from build123d import *

# Parameters (mm, degrees)
F1_DEPTH = 5
F2_D     = 4
F3_R     = 4.9999


# Not quite as in the source:
# - a fillet or chamfer is up to 0.001 mm smaller than in the source, because OpenCascade refuses the exact size
# - ends of sketch curves that miss each other by under 0.0002 mm in the source are joined


with BuildPart() as f1:
    # F0 (on Top) → F1 (new body)
    with BuildSketch(Plane.XY):
        with BuildLine():
            Line((-35, 2.1762e-06), (-35, -35))
            Line((-35, -35), (-27, -35))
            Line((-27, -35), (-27, -22.2710574513))
            ThreePointArc((-27, -22.2710574513), (-32.9393385518, -11.8321585422), (-35, 2.1762e-06))
        make_face()
        with BuildLine():
            Line((-27, -22.2710574513), (-27, -35))
            Line((-27, -35), (0, -35))
            ThreePointArc((0, -35), (-14.9250291324, -31.658229663), (-27, -22.2710574513))
        make_face()
        with BuildLine():
            add(Edge.make_bspline(
                [(0, 45), (-20.1986748725, 45), (-35, 20.0504870868), (-35, 2.1762e-06)],
                knots=[0, 0, 0, 0, 57.0087695372, 57.0087695372, 57.0087695372, 57.0087695372], degree=3))
            ThreePointArc((-35, 2.1762e-06), (-28.4666369261, 20.3629708568), (-11.3056830814, 33.1237306181))
            add(Edge.make_bspline(
                [(0, 37), (-0.2833414452, 37.0069688983), (-1.1232932293, 37.0068386903), (-2.7957299856, 36.8864035146), (-4.9942322029, 36.3521195303), (-7.6997383876, 35.2871018647), (-9.7958540485, 34.148638444), (-11.0540635502, 33.3003360386), (-11.3056830814, 33.1237306181)],
                knots=[0, 0, 0, 0, 0.8506820357, 2.5185967411, 5.0181648841, 7.6012051941, 11.2266191262, 12.1476935207, 12.1476935207, 12.1476935207, 12.1476935207], degree=3))
            add(Edge.make_bspline(
                [(0, 37), (0.2833414452, 37.0069688983), (1.1232932293, 37.0068386903), (2.7957299856, 36.8864035146), (4.9942322029, 36.3521195303), (7.6997383876, 35.2871018647), (9.7958540485, 34.148638444), (11.0540635502, 33.3003360386), (11.3056830814, 33.1237306181)],
                knots=[0, 0, 0, 0, 0.8506820357, 2.5185967411, 5.0181648841, 7.6012051941, 11.2266191262, 12.1476935207, 12.1476935207, 12.1476935207, 12.1476935207], degree=3))
            ThreePointArc((11.3056830814, 33.1237306181), (28.4666375592, 20.3629699719), (35, 0))
            add(Edge.make_bspline(
                [(0, 45), (20.1986748725, 45), (35, 20.0504870868), (35, 0)],
                knots=[0, 0, 0, 0, 57.0087695372, 57.0087695372, 57.0087695372, 57.0087695372], degree=3))
        make_face()
        with BuildLine():
            ThreePointArc((-11.3056830814, 33.1237306181), (-28.4666369261, 20.3629708568), (-35, 2.1762e-06))
            ThreePointArc((-35, 2.1762e-06), (-32.9393385518, -11.8321585422), (-27, -22.2710574513))
            Line((-27, -22.2710574513), (-27, 2.1762e-06))
            add(Edge.make_bspline(
                [(-11.3056830814, 33.1237306181), (-12.4097508436, 32.3488132243), (-15.1414824386, 30.0752135158), (-18.8876274503, 25.5283101279), (-22.422035633, 19.604279738), (-25.0662594291, 13.1120426553), (-26.6478130576, 7.1844788974), (-27.0173066601, 2.7756083867), (-27.018694794, 0.6711028041), (-27, 2.1762e-06)],
                knots=[12.1476935207, 12.1476935207, 12.1476935207, 12.1476935207, 16.189226149, 22.7543847852, 29.7183326598, 36.8091409701, 43.7289829573, 48.0262708445, 50.0404462243, 50.0404462243, 50.0404462243, 50.0404462243], degree=3))
        make_face()
        with BuildLine():
            ThreePointArc((27, -22.2710574513), (14.9250291324, -31.658229663), (0, -35))
            Line((0, -35), (27, -35))
            Line((27, -35), (27, -22.2710574513))
        make_face()
        with BuildLine():
            ThreePointArc((-27, -22.2710574513), (-14.9250291324, -31.658229663), (0, -35))
            ThreePointArc((0, -35), (14.9250291324, -31.658229663), (27, -22.2710574513))
            Line((27, -22.2710574513), (27, 2.1762e-06))
            add(Edge.make_bspline(
                [(11.3056830814, 33.1237306181), (12.4097508436, 32.3488132243), (15.1414824386, 30.0752135158), (18.8876274503, 25.5283101279), (22.422035633, 19.604279738), (25.0662594291, 13.1120426553), (26.6478130576, 7.1844788974), (27.0173066601, 2.7756083867), (27.018694794, 0.6711028041), (27, 2.1762e-06)],
                knots=[12.1476935207, 12.1476935207, 12.1476935207, 12.1476935207, 16.189226149, 22.7543847852, 29.7183326598, 36.8091409701, 43.7289829573, 48.0262708445, 50.0404462243, 50.0404462243, 50.0404462243, 50.0404462243], degree=3))
            ThreePointArc((11.3056830814, 33.1237306181), (0, 35), (-11.3056830814, 33.1237306181))
            add(Edge.make_bspline(
                [(-11.3056830814, 33.1237306181), (-12.4097508436, 32.3488132243), (-15.1414824386, 30.0752135158), (-18.8876274503, 25.5283101279), (-22.422035633, 19.604279738), (-25.0662594291, 13.1120426553), (-26.6478130576, 7.1844788974), (-27.0173066601, 2.7756083867), (-27.018694794, 0.6711028041), (-27, 2.1762e-06)],
                knots=[12.1476935207, 12.1476935207, 12.1476935207, 12.1476935207, 16.189226149, 22.7543847852, 29.7183326598, 36.8091409701, 43.7289829573, 48.0262708445, 50.0404462243, 50.0404462243, 50.0404462243, 50.0404462243], degree=3))
            Line((-27, 2.1762e-06), (-27, -22.2710574513))
        make_face()
        with BuildLine():
            Line((27, -22.2710574513), (27, -35))
            Line((27, -35), (35, -35))
            Line((35, -35), (35, 0))
            ThreePointArc((35, 0), (32.939338184, -11.8321595662), (27, -22.2710574513))
        make_face()
        with BuildLine():
            Line((27, 2.1762e-06), (27, -22.2710574513))
            ThreePointArc((27, -22.2710574513), (32.939338184, -11.8321595662), (35, 0))
            ThreePointArc((35, 0), (28.4666375592, 20.3629699719), (11.3056830814, 33.1237306181))
            add(Edge.make_bspline(
                [(11.3056830814, 33.1237306181), (12.4097508436, 32.3488132243), (15.1414824386, 30.0752135158), (18.8876274503, 25.5283101279), (22.422035633, 19.604279738), (25.0662594291, 13.1120426553), (26.6478130576, 7.1844788974), (27.0173066601, 2.7756083867), (27.018694794, 0.6711028041), (27, 2.1762e-06)],
                knots=[12.1476935207, 12.1476935207, 12.1476935207, 12.1476935207, 16.189226149, 22.7543847852, 29.7183326598, 36.8091409701, 43.7289829573, 48.0262708445, 50.0404462243, 50.0404462243, 50.0404462243, 50.0404462243], degree=3))
        make_face()
        with BuildLine():
            add(Edge.make_bspline(
                [(0, 37), (-0.2833414452, 37.0069688983), (-1.1232932293, 37.0068386903), (-2.7957299856, 36.8864035146), (-4.9942322029, 36.3521195303), (-7.6997383876, 35.2871018647), (-9.7958540485, 34.148638444), (-11.0540635502, 33.3003360386), (-11.3056830814, 33.1237306181)],
                knots=[0, 0, 0, 0, 0.8506820357, 2.5185967411, 5.0181648841, 7.6012051941, 11.2266191262, 12.1476935207, 12.1476935207, 12.1476935207, 12.1476935207], degree=3))
            ThreePointArc((-11.3056830814, 33.1237306181), (0, 35), (11.3056830814, 33.1237306181))
            add(Edge.make_bspline(
                [(0, 37), (0.2833414452, 37.0069688983), (1.1232932293, 37.0068386903), (2.7957299856, 36.8864035146), (4.9942322029, 36.3521195303), (7.6997383876, 35.2871018647), (9.7958540485, 34.148638444), (11.0540635502, 33.3003360386), (11.3056830814, 33.1237306181)],
                knots=[0, 0, 0, 0, 0.8506820357, 2.5185967411, 5.0181648841, 7.6012051941, 11.2266191262, 12.1476935207, 12.1476935207, 12.1476935207, 12.1476935207], degree=3))
        make_face()
    extrude(amount=F1_DEPTH)

    # F2 (through all)
    with Locations(Plane(origin=(0, 0, 0), x_dir=(1, 0, 0), z_dir=(0, 0, -1))):
        with Locations((0, -37), (-7.7739062126, -35.111513252), (-14.2579257305, -30.4256311694), (-19.3371352018, -24.244884358), (-23.1543015859, -17.2142911543), (-25.7431047524, -9.6447404302), (-26.9552512695, -1.7371048277), (-27, 6.2627700182), (-27, 14.2627700182), (-27, 22.2627700182), (7.7739062126, -35.111513252), (14.2579257305, -30.4256311694), (19.3371352018, -24.244884358), (23.1543015859, -17.2142911543), (25.7431047524, -9.6447404302), (26.9552512695, -1.7371048277), (27, 6.2627700182), (27, 14.2627700182), (27, 22.2627700182)):
            Hole(F2_D / 2)

    # F3 (radius 5 in the source; OpenCascade refuses exactly that, so slightly less here)
    f3_edges = [f1.edges().sort_by_distance(p)[0] for p in [
        (-35, -35, 2.5),
        (35, -35, 2.5),
        (-35, -17.499999, 5),
        (0, -35, 5),
    ]]
    fillet(f3_edges, radius=F3_R)


solid = f1.part
Part model, mm, in its own coordinate system. Give positions to 0.01 mm unless a question says otherwise; leave off trailing zeros. Put each result on its own line as item: value. Start each with the question number.
1) Saw through at B-B (z = 1.9). State how many separate pieces and enclosed holes the cut face has, then the cut area to 3 significant figures.
2) Pull direction X, two halves, no side cores. Call faces 1 (the cylindrical face through (-33, -15, 4)), 2 (the cylindrical face through (-28.91, -6.86, 2.53)), 3 (the cylindrical face through (0, -34, 3)): +X half, -X half, draft (parallel to the pull), parting line (faces both ways), or undercut.
3) Flat gauge pins, fed straight in: pin 1 (1.5 mm diameter, centred on x = -3, z = 2.5, fed in from -Y); pin 2 (3 mm diameter, centred on x = 15.5, z = 3.5, fed in from -Y); pin 3 (3 mm diameter, centred on y = 5, z = 1, fed in from -X). Where does each tip first touch, or does it go through?
4) Probe probe 1 along Y at (x, z) = (-28.5, 0.8); probe 2 along X at (y, z) = (23, 4.2); probe 3 along X at (y, z) = (11, 1). List the from-to ranges inside material, lowest first.
Numbers:
1. separate pieces: 1
1. enclosed holes: 19
1. area: 4,520 mm^2
2. face 1: -X half
2. face 2: undercut
2. face 3: draft
3. pin 1: y = -34.68
3. pin 2: y = -34.58
3. pin 3: x = -34.83
4. probe 1: -34.94 to -23.59, -20.94 to -15.59, -12.94 to -7.59, -4.94 to 0.47, 3.01 to 24.36
4. probe 2: -26.71 to -20.9, -17.77 to 17.77, 20.9 to 26.71
4. probe 3: -33.54 to -27.21, -24.27 to 24.27, 27.21 to 33.54
